Can you work these out from the model? Positions are in its coordinate system, mm. Round coordinates to 2 decimals unless told otherwise and drop trailing zeros. Loops run counter-clockwise (first coordinate to the right, second up) from the corner with the lowest first, then second, coordinate; pieces in that order, holes last.
Autodesk Inventor part; units mm, degrees
ref_plane "YZ Plane" through (0, 0, 0) normal (1, 0, 0) x (0, 1, 0)
ref_plane "XZ Plane" through (0, 0, 0) normal (0, 1, 0) x (-1, 0, 0)
ref_plane "XY Plane" through (0, 0, 0) normal (0, 0, 1) x (1, 0, 0)
sketch "Sketch1" plane through (0, 0, 0) normal (0, 0, 1) x (1, 0, 0)
  line L0 (0, 0) -> (50.8, 0)
  line L1 (50.8, 0) -> (50.8, 169.8752)
  line L2 (50.8, 169.8752) -> (0, 169.8752)
  line L3 (0, 169.8752) -> (0, 0)
  line L4 (25.4, 169.8752) -> (25.4, 144.4752)
  line L5 (25.4, 169.8752) -> (50.8, 169.8752) construction
  circle A0 centre (25.4, 144.4752) radius 14.2875
  line L6 (25.4, 144.4752) -> (43.3605, 162.4357)
  line L7 (25.4, 144.4752) -> (50.8, 144.4752) construction
  line L8 (7.4395, 126.5147) -> (43.3605, 126.5147)
  line L9 (43.3605, 162.4357) -> (7.4395, 162.4357)
  line L10 (7.4395, 162.4357) -> (7.4395, 126.5147)
  circle A1 centre (7.4395, 162.4357) radius 2.032
  circle A2 centre (7.4395, 126.5147) radius 2.032
  circle A3 centre (43.3605, 162.4357) radius 2.032
  circle A4 centre (43.3605, 126.5147) radius 2.032
  line L11 (0, 0) -> (50.8, 0)
  line L12 (50.8, 0) -> (50.8, 38.1)
  line L13 (0, 38.1) -> (0, 0)
  line L14 (25.4, 38.1) -> (12.7, 38.1)
  line L15 (25.4, 38.1) -> (38.1, 38.1) construction
  line L16 (12.7, 38.1) -> (38.1, 38.1)
  circle A5 centre (12.7, 38.1) radius 3.175
  circle A6 centre (38.1, 38.1) radius 3.175
  dimension "d0" = 50.8
  dimension "d1" = 169.8752
  dimension "d2" = 25.4
  dimension "d3" = 90
  dimension "d4" = 28.575
  dimension "d5" = 25.4
  dimension "d6" = 45
  dimension "d7" = 50.8
  dimension "d9" = 4.064
  dimension "d10" = 4.064
  dimension "d11" = 4.064
  dimension "d12" = 4.064
  dimension "d13" = 50.8
  dimension "d14" = 38.1
  dimension "d15" = 12.7
  dimension "d16" = 180
  dimension "d17" = 25.4
  dimension "d18" = 0
  dimension "d19" = 6.35
  dimension "d20" = 6.35
extrude "Extrusion1" add sketch "Sketch1" along normal blind 25.4 contours L9 A3 L6 A0 L4 | L3 L2 L1 L0
sketch "Sketch2" plane through (0, 169.8752, 0) normal (0, 1, 0) x (1, 0, 0)
  line L0 (0, 0) -> (3.175, 0)
  line L1 (3.175, 0) -> (3.175, -3.175)
  line L2 (3.175, -3.175) -> (0, -3.175)
  line L3 (0, -3.175) -> (0, 0)
  line L4 (3.175, -3.175) -> (47.625, -3.175)
  line L5 (47.625, -3.175) -> (47.625, -22.225)
  line L6 (47.625, -22.225) -> (3.175, -22.225)
  line L7 (3.175, -22.225) -> (3.175, -3.175)
  dimension "d23" = 3.175
  dimension "d24" = 3.175
  dimension "d25" = 44.45
  dimension "d26" = 19.05
extrude "Extrusion2" cut sketch "Sketch2" against normal blind 254 contours L4 L5 L6 L7
sketch "Sketch3" plane through (0, 0, 25.4) normal (0, 0, 1) x (1, 0, 0)
  circle A0 centre (12.7, 38.1) radius 3.175
  line L0 (12.7, 38.1) -> (38.1, 38.1)
  line L1 (38.1, 38.1) -> (38.1, 12.7)
  line L2 (38.1, 12.7) -> (12.7, 12.7)
  line L3 (12.7, 12.7) -> (12.7, 38.1)
  circle A1 centre (12.7, 12.7) radius 3.175
  circle A2 centre (38.1, 12.7) radius 3.175
  dimension "d29" = 25.4
  dimension "d30" = 25.4
  dimension "d31" = 6.35
  dimension "d32" = 6.35
extrude "Extrusion3" cut sketch "Sketch3" against normal blind 25.4 contours A1 L2 L3 | L3 L2 A1 | A2 L2 L1 | L1 L2 A2
sketch "Sketch4" plane through (0, 169.8752, 0) normal (0, 1, 0) x (1, 0, 0)
  line L0 (47.625, -22.225) -> (3.175, -22.225)
  line L1 (3.175, -22.225) -> (3.175, -3.175)
  line L2 (3.175, -3.175) -> (47.625, -3.175)
  line L3 (47.625, -3.175) -> (47.625, -22.225)
  line L4 (50.8, 0) -> (50.8, -25.4)
  line L5 (0, 0) -> (50.8, 0)
  line L6 (50.8, 0) -> (50.8, -22.225)
  line L7 (50.8, -22.225) -> (0, -22.225)
  line L8 (0, -22.225) -> (0, 0)
extrude "Extrusion4" cut sketch "Sketch4" against normal blind 254 contours L3 L2 L1 L7 L8 L5 L4
sketch "Sketch5" plane through (0, 0, 25.4) normal (0, 0, 1) x (1, 0, 0)
  circle A0 centre (38.1, 12.7) radius 3.175
  circle A1 centre (12.7, 12.7) radius 3.175
  circle A2 centre (25.4, 144.4752) radius 14.2875
  circle A3 centre (38.1, 38.1) radius 3.175
  circle A4 centre (12.7, 38.1) radius 3.175
  circle A5 centre (43.3605, 126.5147) radius 2.032
  circle A6 centre (43.3605, 162.4357) radius 2.032
  circle A7 centre (7.4395, 126.5147) radius 2.032
  circle A8 centre (7.4395, 162.4357) radius 2.032
  line L0 (0, 0) -> (50.8, 0)
  line L1 (50.8, 0) -> (50.8, 169.8752)
  line L2 (50.8, 169.8752) -> (0, 169.8752)
  line L3 (0, 169.8752) -> (0, 0)
extrude "Extrusion5" add sketch "Sketch5" along normal blind 3.175
sketch "Sketch6" plane through (0, 0, 28.575) normal (0, 0, 1) x (1, 0, 0)
  circle A0 centre (25.4, 144.4752) radius 14.2875
  circle A1 centre (25.4, 144.4752) radius 9.525
  dimension "d39" = 19.05
extrude "Extrusion6" add sketch "Sketch6" against normal blind 6.35
sketch "Sketch7" plane through (0, 0, 28.575) normal (0, 0, 1) x (1, 0, 0)
  line L0 (50.8, 169.8752) -> (0, 169.8752)
  line L1 (0, 169.8752) -> (0, 0)
  line L2 (25.4, 169.8752) -> (25.4, 95.25)
  line L3 (25.4, 169.8752) -> (100.0252, 169.8752) construction
  circle A0 centre (25.4, 95.25) radius 7.9375
  dimension "d43" = 74.6252
  dimension "d44" = 90
  dimension "d45" = 15.875
extrude "Extrusion7" cut sketch "Sketch7" against normal blind 25.4
sketch "Sketch8" plane through (0, 0, 28.575) normal (0, 0, 1) x (1, 0, 0)
  circle A0 centre (25.4, 144.4752) radius 9.525
  circle A1 centre (25.4, 144.4752) radius 14.2875
  dimension "d48" = 28.575
extrude "Extrusion8" cut sketch "Sketch8" against normal blind 25.4
sketch "Sketch9" plane through (0, 0, 28.575) normal (0, 0, 1) x (1, 0, 0)
  circle A0 centre (25.4, 95.25) radius 7.9375
  circle A1 centre (7.4395, 162.4357) radius 2.032
  circle A2 centre (7.4395, 126.5147) radius 2.032
  circle A3 centre (43.3605, 162.4357) radius 2.032
  circle A4 centre (43.3605, 126.5147) radius 2.032
  line L0 (25.4, 95.25) -> (43.3605, 113.2105)
  line L1 (25.4, 95.25) -> (50.8, 95.25) construction
  line L2 (43.3605, 113.2105) -> (7.4395, 77.2895)
  circle A5 centre (7.4395, 113.2105) radius 2.032
  circle A6 centre (43.3605, 113.2105) radius 2.032
  circle A7 centre (43.3605, 77.2895) radius 2.032
  circle A8 centre (7.4395, 77.2895) radius 2.032
  dimension "d51" = 25.4
  dimension "d52" = 45
  dimension "d53" = 50.8
  dimension "d54" = 0
  dimension "d55" = 4.064
  dimension "d56" = 4.064
  dimension "d57" = 4.064
  dimension "d58" = 4.064
extrude "Extrusion9" cut sketch "Sketch9" against normal blind 6.35 contours A8 | A6 | A1 | A2 | A3 | A4 | A5 | A7
sketch "Sketch10" plane through (0, 0, 28.575) normal (0, 0, 1) x (1, 0, 0)
  circle A0 centre (7.4395, 162.4357) radius 2.032
  circle A1 centre (7.4395, 126.5147) radius 2.032
  circle A2 centre (43.3605, 162.4357) radius 2.032
  circle A3 centre (43.3605, 126.5147) radius 2.032
extrude "Extrusion10" add sketch "Sketch10" against normal blind 6.35
properties part number "Z-Plate"
(1) For pin 1 (5 mm diameter, centred on x = 38.1, y = 38.1, fed in from -Z), with a flat end and sliding along its axis, tell me the tip position at first contact or that it passes through.
(2) We'd pull the mould along Y, two halves only. Please class faces 1 (the flat face through (25, 0, 25)), 2 (the flat face through (25, 86, 22.225)), 3 (the cylindrical face through (35.76, 35.954, 25.356)), 4 (the flat face through (26, 169.875, 25)): released by +Y, released by -Y, zero draft, split by the parting line, or undercut.
(3) Suppose I cut it at B-B (y = 95.25). Write out the boundary of the cut face in (x, z) (1 decimal).
(4) If I drill on line 1 (Y direction, x = 43.5, z = 26.75); line 2 (X direction, y = 38.1, z = 25) (3 decimals); line 3 (Y direction, x = 25.5, z = 24), over which ranges is the centre line in solid material (lowest first)?
(5) Suppose I cut it at D-D (x = 37). Write out the boundary of the cut face in (y, z) (3 decimals).
(6) Suppose I cut it at C-C (y = 12.7). Write out the boundary of the cut face in (x, z) (3 decimals), then the cut area to 3 significant figures.
(7) Suppose I cut it at A-A (x = 25.4). Write out the boundary of the cut face in (y, z) (1 decimal), then the cut area to 3 significant figures.
Check result:
1. pin 1: passes through
2. face 1: released by -Y
2. face 2: zero draft
2. face 3: undercut
2. face 4: released by +Y
3. outline: (0, 22.2) - (17.5, 22.2) - (17.5, 28.6) - (0, 28.6) - close; (33.3, 22.2) - (50.8, 22.2) - (50.8, 28.6) - (33.3, 28.6) - close
4. line 1: y = 0 to 75.26, 79.32 to 111.18, 115.24 to 169.88
4. line 2: x = 0 to 9.525, 15.875 to 34.925, 41.275 to 50.8
4. line 3: y = 0 to 87.31, 103.19 to 130.19, 158.76 to 169.88
5. outline: (0, 22.225) - (9.722, 22.225) - (9.722, 28.575) - (0, 28.575) - close; (15.678, 22.225) - (35.122, 22.225) - (35.122, 28.575) - (15.678, 28.575) - close; (41.078, 22.225) - (136.134, 22.225) - (136.134, 28.575) - (41.078, 28.575) - close; (152.816, 22.225) - (169.875, 22.225) - (169.875, 28.575) - (152.816, 28.575) - close
6. outline: (0, 22.225) - (9.525, 22.225) - (9.525, 28.575) - (0, 28.575) - close; (15.875, 22.225) - (34.925, 22.225) - (34.925, 28.575) - (15.875, 28.575) - close; (41.275, 22.225) - (50.8, 22.225) - (50.8, 28.575) - (41.275, 28.575) - close
6. area: 242 mm2
7. outline: (0, 22.2) - (87.3, 22.2) - (87.3, 28.6) - (0, 28.6) - close; (103.2, 22.2) - (130.2, 22.2) - (130.2, 28.6) - (103.2, 28.6) - close; (158.8, 22.2) - (169.9, 22.2) - (169.9, 28.6) - (158.8, 28.6) - close
7. area: 796 mm2
